Verification items for the finished model (mm, model axes). A direction names the side the tool comes from. Coordinates: 2 decimals unless noted, no trailing zeros. Order: outer loops, then holes, each group sorted by start corner. A loop starts at its lowest first (then second) coordinate and runs counter-clockwise, first axis right, second up. Notation, with made-up numbers: (29, -40) -> (84, -40) arc R27 cw to (84, -1) -> close; hole circle Ø1 at (17.5, -29.5). An arc over 180 degrees is marked (long way). Write item = value, one per line. Start each with the question number.
from build123d import *

# Parameters (mm, degrees)
F0_W     = 2286
F0_H     = 1270
F1_DEPTH = 635
F2_W     = 1016
F2_H     = 1270
F3_DEPTH = 381
F5_DEPTH = 635


with BuildPart() as f1:
    # F0 (on Front) → F1 (new body)
    with BuildSketch(Plane.XZ):
        with Locations((1143, 635)):
            Rectangle(F0_W, F0_H)
    extrude(amount=F1_DEPTH)

    # F2 (on face) → F3 (cut)
    with BuildSketch(Plane.XZ.offset(635)):
        with Locations((1143, 635)):
            Rectangle(F2_W, F2_H)
    extrude(amount=-F3_DEPTH, mode=Mode.SUBTRACT)

    # F4 (on face) → F5 (cut)
    with BuildSketch(Plane(origin=(0, 0, 0), x_dir=(-1, 0, 0), z_dir=(0, 1, 0))):
        Polygon((-1143, 381), (-381, 1270), (-2286, 1270), (-2286, 1016), (-1905, 1016), align=None)
    extrude(amount=-F5_DEPTH, mode=Mode.SUBTRACT)


solid = f1.part
Item 1: Thickness scan on line 1 (X direction, y = -264, z = 557.5); line 2 (Y direction, x = 910.5, z = 342.5); line 3 (Z direction, x = 2089, y = -229). Record the ranges inside material, lowest first.
Item 2: Tool access check on faces 4 (the flat face through (1127, -242, 0)), 5 (the flat face through (682.67, -242.5, 918.05)), 6 (the flat face through (1136, -254, 385)). Record the directions out of +Z, -Z, +X, -X, +Y, -Y that give a thin tool (end or side, any length) a straight path to the whole face; none if there is none.
Item 3: Section check D-D (y = -205). Record the boundary of the cut face in (x, z).
Item 4: Section check B-B (z = 874). Record the boundary of the cut face in (x, y).
Item 5: Section check C-C (z = 328). Record the boundary of the cut face in (x, y), then the cut area to 3 significant figures.
Item 6: Mould release check, pull along X, two halves, no side actions. Record for faces 1 (the flat face through (1614, -242.5, 773.5)), 2 (the flat face through (2098, -313, 1016)), 3 (the flat face through (0, -313, 626)): pulls with the +X half, pulls with the -X half, needs draft (parallel to the pull), parting line crosses it, or undercut.
Item 7: Section check A-A (y = -535). Record the boundary of the cut face in (x, z), then the cut area to 3 significant figures.
Filled sheet:
q1.line_1 = 0 to 635, 1651 to 2286
q1.line_2 = -254 to 0
q1.line_3 = 0 to 1016
q2.face_4 = -Z, +X, -X, +Y, -Y
q2.face_5 = +Z, +Y, -Y
q2.face_6 = +Z, -Z, -Y
q3.outline = (0, 0) -> (2286, 0) -> (2286, 1016) -> (1905, 1016) -> (1143, 381) -> (381, 1270) -> (0, 1270) -> close
q4.outline = (0, -635) -> (635, -635) -> (635, -254) -> (720.43, -254) -> (720.43, 0) -> (0, 0) -> close; (1734.6, -635) -> (2286, -635) -> (2286, 0) -> (1734.6, 0) -> close
q5.outline = (0, -635) -> (635, -635) -> (635, -254) -> (1651, -254) -> (1651, -635) -> (2286, -635) -> (2286, 0) -> (0, 0) -> close
q5.area = 1,060,000 mm^2
q6.face_1 = undercut
q6.face_2 = needs draft
q6.face_3 = pulls with the -X half
q7.outline = (0, 0) -> (635, 0) -> (635, 973.67) -> (381, 1270) -> (0, 1270) -> close; (1651, 0) -> (2286, 0) -> (2286, 1016) -> (1905, 1016) -> (1651, 804.33) -> close
q7.area = 1,390,000 mm^2
